Design review of the part built by this model. Coordinates are the model's own, in mm. A direction names the side the tool comes from. Coordinates: 2 decimals unless noted, no trailing zeros. Loops run counter-clockwise (first coordinate to the right, second up) from the corner with the lowest first, then second, coordinate; pieces in that order, holes last. Notation, with made-up numbers: (84.5, 57) -> (90.5, 57) arc R35 cw to (90.5, 90) -> close; hole circle Ø5 at (53.5, -14). An arc over 180 degrees is marked (long way). Answer in a Markdown table with one row per item.
```python
from build123d import *

# Parameters (mm, degrees)
ESQUISSE1_W                = 100
ESQUISSE1_H                = 15
BOSS_EXTRU_1_DEPTH         = 80
BOSS_EXTRU_1_TAPER         = 2.5
ESQUISSE2_W                = 1
ESQUISSE2_H                = 2.5
ENL_V_MAT_EXTRU_1_DEPTH    = 127.859596195
ENL_V_MAT_EXTRU_2_DEPTH    = 2
ESQUISSE5_R                = 1
R_P_TITION_LIN_AIRE1_COUNT = 3
R_P_TITION_LIN_AIRE1_PITCH = 38
CONG_1_R                   = 0.8
CONG_2_R                   = 0.8


with BuildPart() as part:
    # Esquisse1 → Boss.-Extru.1 (new body)
    with BuildSketch(Plane.XY):
        Rectangle(ESQUISSE1_W, ESQUISSE1_H)
    extrude(amount=BOSS_EXTRU_1_DEPTH, taper=BOSS_EXTRU_1_TAPER)

    # Esquisse2 → Enlèv. mat.-Extru.1 (cut, through all)
    with BuildSketch(Plane(origin=(49.904867452, 0, 2.178893569), x_dir=(0.043619387365336104, 0, -0.9990482215818578), z_dir=(0.9990482215818577, 0, 0.0436193873653361))):
        with Locations((1.680969368, 0)):
            Rectangle(ESQUISSE2_W, ESQUISSE2_H)
    enl_v_mat_extru_1 = extrude(amount=-ENL_V_MAT_EXTRU_1_DEPTH, mode=Mode.SUBTRACT)

    # Symétrie1: Enlèv. mat.-Extru.1 across plane
    add(enl_v_mat_extru_1.mirror(Plane(origin=(0, 0, 0), x_dir=(0, 0, 1), z_dir=(1, 0, 0))), mode=Mode.SUBTRACT)

    # Esquisse3 → Enlèv. mat.-Extru.2 (cut)
    with BuildSketch(Plane(origin=(0, 7.485730118, 0.326834035), x_dir=(1, 0, 0), z_dir=(0, 0.9990482215818577, 0.0436193873653361))):
        Polygon((53.133710782, 3.327145405), (-53.133710782, 3.327145405), (-49.379119025, -82.749069408), (49.379119025, -82.749069408), align=None)
        Polygon((46.866289218, -2.672854595), (-46.866289218, -2.672854595), (-43.635130109, -76.749069408), (43.635130109, -76.749069408), align=None, mode=Mode.SUBTRACT)
    enl_v_mat_extru_2 = extrude(amount=-ENL_V_MAT_EXTRU_2_DEPTH, mode=Mode.SUBTRACT)

    # Symétrie2: Enlèv. mat.-Extru.2 across plane
    add(enl_v_mat_extru_2.mirror(Plane.ZX), mode=Mode.SUBTRACT)

    # Balayage1: sweep along a path in Esquisse4
    with BuildLine(Plane(origin=(0, -3.347747388, 76.6760213), x_dir=(1, 0, 0), z_dir=(0, -0.043619387365336104, 0.9990482215818578))) as balayage1_path:
        Line((-37.620500895, 5.492861662), (-37.620500895, 35.492861662))
    # Esquisse5 → Balayage1 (sweep)
    with BuildSketch(Plane(origin=(0, 5.487633675, 0.239595261), x_dir=(1, 0, 0), z_dir=(0, 0.9990482215818578, 0.04361938736533611))):
        with Locations((-37.691661974, -78.336391294)):
            Circle(ESQUISSE5_R)
    balayage1 = sweep(path=balayage1_path.line)

    # Répétition linéaire1: Balayage1 ×3
    with Locations(*[(i * R_P_TITION_LIN_AIRE1_PITCH, 0, 0) for i in range(1, R_P_TITION_LIN_AIRE1_COUNT)]):
        add(balayage1)

    # Congé1
    cong_1_edges = [part.edges().sort_by_distance(p)[0] for p in [
        (-38.691661974, 32.042094925, 79.810009289),
        (-0.691661974, 32.042094925, 79.810009289),
        (37.308338026, 32.042094925, 79.810009289),
    ]]
    fillet(cong_1_edges, radius=CONG_1_R)

    # Congé2
    cong_2_edges = [part.edges().sort_by_distance(p)[0] for p in [
        (0, 2.005219197, 80),
        (0, 5.49809463, 0),
        (-48.253562284, 3.751656913, 40),
        (48.253562284, 3.751656913, 40),
        (45.250709663, 5.753562284, 40),
        (0, 4.137982729, 77.002855335),
        (-45.250709663, 5.753562284, 40),
        (0, 7.369141838, 2.997144665),
    ]]
    fillet(cong_2_edges, radius=CONG_2_R)


solid = part.part
```
(1) Draft analysis for pull direction Y (two halves, no side actions). For faces 1 (the flat face through (-1, 0, 0)), 2 (the flat face through (-38.676, -0.017, 0.507)), 3 (the flat face through (0.656, -5.776, 39.482)), state which applies: pulls with the +Y half, pulls with the -Y half, needs draft (parallel to the pull), parting line crosses it, or undercut.
Evaluation:
| item | result |
|---|---|
| face 1 | needs draft |
| face 2 | undercut |
| face 3 | pulls with the -Y half |
(2) Tool access review of faces 4 (the flat face through (-48.666, -0.471, 30.551)), 5 (the flat face through (38.676, -0.017, 0.507)): name each direction out of +Z, -Z, +X, -X, +Y, -Y from which nothing blocks a thin tool from reaching the whole face with its end or side.
Evaluation:
| item | result |
|---|---|
| face 4 | +Z, -X, +Y, -Y |
| face 5 | -Z, +X |
(3) To check wall thickness, follow probe 1 along Z at (x, y) = (19, 0.5); probe 2 along Z at (x, y) = (-9.5, -2.5); probe 3 along Y at (x, z) = (37, 60.5). State the ranges of each line that lie inside material, in increasing order.
Evaluation:
| item | result |
|---|---|
| probe 1 | z = 0 to 80 |
| probe 2 | z = 0 to 76.93 |
| probe 3 | y = -4.86 to 4.86 |
(4) Take a section at A-A on x = -7.5. Give the boundary of the cut face in (y, z) (3 decimals), and give its area (3 significant figures).
Evaluation:
| item | result |
|---|---|
| outline | (-7.369, 2.997) -> (-5.371, 2.91) -> (-5.498, 0) -> (4.662, 0) arc R0.8 ccw to (5.462, 0.835) -> (5.371, 2.91) -> (6.57, 2.962) arc R0.8 ccw to (7.334, 3.796) -> (4.173, 76.204) arc R0.8 ccw to (3.339, 76.968) -> (2.14, 76.916) -> (2.039, 79.235) arc R0.8 ccw to (1.239, 80) -> (-2.005, 80) -> (-2.14, 76.916) -> (-4.138, 77.003) -> close |
| area | 896 mm² |
(5) For pin 1 (1.5 mm diameter, centred on x = 30, z = 21.5, fed in from -Y); pin 2 (12 mm diameter, centred on y = 0.5, z = 21.5, fed in from +X); pin 3 (8 mm diameter, centred on x = 38.5, z = 67, fed in from -Y), all flat-tipped, find the tip position at first contact; note any pin that passes through.
Evaluation:
| item | result |
|---|---|
| pin 1 | stops at y = -6.59 |
| pin 2 | stops at x = 49.32 |
| pin 3 | stops at y = -4.75 |
(6) Take a section at C-C on y = 26. Count the separate pieces of the cut face and the enclosed holes in it, and give its area (3 significant figures).
Evaluation:
| item | result |
|---|---|
| separate pieces | 3 |
| enclosed holes | 0 |
| area | 9.43 mm² |
(7) Take a section at B-B on x = 41. Give the boundary of the cut face in (y, z) (3 decimals), and give its area (4 significant figures).
Evaluation:
| item | result |
|---|---|
| outline | (-7.369, 2.997) -> (-5.371, 2.91) -> (-5.498, 0) -> (-1.25, 0) -> (-1.25, 0.608) -> (1.25, 0.608) -> (1.25, 0) -> (4.662, 0) arc R0.8 ccw to (5.462, 0.835) -> (5.371, 2.91) -> (6.57, 2.962) arc R0.8 ccw to (7.334, 3.796) -> (4.173, 76.204) arc R0.8 ccw to (3.339, 76.968) -> (2.14, 76.916) -> (2.039, 79.235) arc R0.8 ccw to (1.239, 80) -> (-2.005, 80) -> (-2.14, 76.916) -> (-4.138, 77.003) -> close |
| area | 894.5 mm² |
